Source: CAD feature listing. Evaluate the final solid. Frame: model axes, mm. Coordinates: 2 decimals unless noted, no trailing zeros. Order: outer loops, then holes, each group sorted by start corner. A loop starts at its lowest first (then second) coordinate and runs counter-clockwise, first axis right, second up.
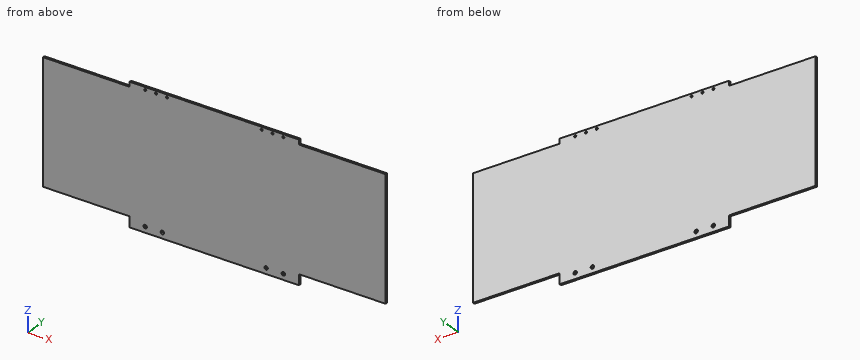
```python
from build123d import *

# Parameters (mm, degrees)
SKETCH1_R           = 2.564
SKETCH1_R_2         = 1.54
BOSS_EXTRUDE1_DEPTH = 3


with BuildPart() as part:
    # Sketch1 → Boss-Extrude1 (new body)
    with BuildSketch(Plane(origin=(0, 0, 0), x_dir=(1, 0, 0), z_dir=(0, 1, 0))):
        Polygon((128, 0), (128, -7), (378, -7), (378, 0), (506, 0), (506, 180), (378, 180), (378, 195.398), (128, 195.398), (128, 180), (0, 180), (0, 0), align=None)
        with Locations(Location((151, 186.858, 0), (0, 0, 270))):
            Circle(SKETCH1_R, mode=Mode.SUBTRACT)
        with Locations(Location((176.4, 186.858, 0), (0, 0, 270))):
            Circle(SKETCH1_R, mode=Mode.SUBTRACT)
        with Locations(Location((151, -3, 0), (0, 0, 270))):
            Circle(SKETCH1_R_2, mode=Mode.SUBTRACT)
        with Locations(Location((183, -3, 0), (0, 0, 270))):
            Circle(SKETCH1_R_2, mode=Mode.SUBTRACT)
        with Locations(Location((329.6, 186.858, 0), (0, 0, 90))):
            Circle(SKETCH1_R, mode=Mode.SUBTRACT)
        with Locations(Location((355, 186.858, 0), (0, 0, 90))):
            Circle(SKETCH1_R, mode=Mode.SUBTRACT)
        with Locations(Location((167, -3, 0), (0, 0, 270))):
            Circle(SKETCH1_R_2, mode=Mode.SUBTRACT)
        with Locations(Location((323, -3, 0), (0, 0, 90))):
            Circle(SKETCH1_R_2, mode=Mode.SUBTRACT)
        with Locations(Location((339, -3, 0), (0, 0, 90))):
            Circle(SKETCH1_R_2, mode=Mode.SUBTRACT)
        with Locations(Location((355, -3, 0), (0, 0, 90))):
            Circle(SKETCH1_R_2, mode=Mode.SUBTRACT)
    extrude(amount=BOSS_EXTRUDE1_DEPTH)


solid = part.part
```
1. Section query B-B, the plane x = 415.5. Output: boundary loops of the cut face in (y, z), plus the area to 3 significant figures.
2. Contact query for flat-ended pins moving along their axis: P1, Ø3.5, axis at x = 183, z = 3, coming from the +Y side; P2, Ø3, axis at x = 151, z = -186.858, coming from the -Y side; P3, Ø0.9, axis at x = 434.5, y = 2, coming from the +Z side; P4, Ø1.5, axis at y = 1.5, z = 2, coming from the +X side. Output: stop coordinate, or through.
3. Material intervals for line 1 along Z through (x, y) = (151, 1.65); line 2 along Z through (x, y) = (176.4, 1.7); line 3 along Z through (x, y) = (394.5, 1.15), sorted ascending.
4. Section query A-A, the plane y = 0.95. Count the separate pieces of the cut face and the enclosed holes in it, plus the area to 3 significant figures.
Answer key:
1. outline: (0, -180) - (3, -180) - (3, 0) - (0, 0) - close
1. area: 540 mm2
2. P1: stops at y = 3
2. P2: passes through
2. P3: stops at z = 0
2. P4: stops at x = 378
3. line 1: z = -195.4 to -189.42, -184.29 to 1.46, 4.54 to 7
3. line 2: z = -195.4 to -189.42, -184.29 to 7
3. line 3: z = -180 to 0
4. separate pieces: 1
4. enclosed holes: 10
4. area: 96,600 mm2
